```python
from build123d import *

# Parameters (mm, degrees)
SKETCH1_W           = 152.4
SKETCH1_H           = 69.85
BOSS_EXTRUDE1_DEPTH = 19.05
CUT_EXTRUDE1_DEPTH  = 7.1374
CUT_EXTRUDE2_REACH  = 71.85
SKETCH3_R           = 4.0132


with BuildPart() as part:
    # Sketch1 → Boss-Extrude1 (new body)
    with BuildSketch(Plane.XY):
        Rectangle(SKETCH1_W, SKETCH1_H)
    extrude(amount=BOSS_EXTRUDE1_DEPTH)

    # Sketch2 → Cut-Extrude1 (cut)
    with BuildSketch(Plane.XY.offset(19.05)):
        with BuildLine():
            Line((-45.24375, 28.575), (-30.95625, 28.575))
            ThreePointArc((-30.95625, 28.575), (-27.588653955, 27.180096045), (-26.19375, 23.8125))
            Line((-26.19375, 23.8125), (-26.19375, -23.8125))
            ThreePointArc((-26.19375, -23.8125), (-27.588653955, -27.180096045), (-30.95625, -28.575))
            Line((-30.95625, -28.575), (-45.24375, -28.575))
            ThreePointArc((-45.24375, -28.575), (-48.611346045, -27.180096045), (-50.00625, -23.8125))
            Line((-50.00625, -23.8125), (-50.00625, 23.8125))
            ThreePointArc((-50.00625, 23.8125), (-48.611346045, 27.180096045), (-45.24375, 28.575))
        make_face()
        with BuildLine():
            Line((7.14375, 28.575), (-7.14375, 28.575))
            ThreePointArc((-7.14375, 28.575), (-10.511346045, 27.180096045), (-11.90625, 23.8125))
            Line((-11.90625, 23.8125), (-11.90625, -23.8125))
            ThreePointArc((-11.90625, -23.8125), (-10.511346045, -27.180096045), (-7.14375, -28.575))
            Line((-7.14375, -28.575), (7.14375, -28.575))
            ThreePointArc((7.14375, -28.575), (10.511346045, -27.180096045), (11.90625, -23.8125))
            Line((11.90625, -23.8125), (11.90625, 23.8125))
            ThreePointArc((11.90625, 23.8125), (10.511346045, 27.180096045), (7.14375, 28.575))
        make_face()
        with BuildLine():
            Line((30.95625, 28.575), (45.24375, 28.575))
            ThreePointArc((45.24375, 28.575), (48.611346045, 27.180096045), (50.00625, 23.8125))
            Line((50.00625, 23.8125), (50.00625, -23.8125))
            ThreePointArc((50.00625, -23.8125), (48.611346045, -27.180096045), (45.24375, -28.575))
            Line((45.24375, -28.575), (30.95625, -28.575))
            ThreePointArc((30.95625, -28.575), (27.588653955, -27.180096045), (26.19375, -23.8125))
            Line((26.19375, -23.8125), (26.19375, 23.8125))
            ThreePointArc((26.19375, 23.8125), (27.588653955, 27.180096045), (30.95625, 28.575))
        make_face()
        with BuildLine():
            Line((-69.85, 28.575), (-66.675, 28.575))
            ThreePointArc((-66.675, 28.575), (-64.42993597, 27.64506403), (-63.5, 25.4))
            Line((-63.5, 25.4), (-63.5, -25.4))
            ThreePointArc((-63.5, -25.4), (-64.42993597, -27.64506403), (-66.675, -28.575))
            Line((-66.675, -28.575), (-69.85, -28.575))
            ThreePointArc((-69.85, -28.575), (-72.09506403, -27.64506403), (-73.025, -25.4))
            Line((-73.025, -25.4), (-73.025, 25.4))
            ThreePointArc((-73.025, 25.4), (-72.09506403, 27.64506403), (-69.85, 28.575))
        make_face()
        with BuildLine():
            Line((66.675, 28.575), (69.85, 28.575))
            ThreePointArc((69.85, 28.575), (72.09506403, 27.64506403), (73.025, 25.4))
            Line((73.025, 25.4), (73.025, -25.4))
            ThreePointArc((73.025, -25.4), (72.09506403, -27.64506403), (69.85, -28.575))
            Line((69.85, -28.575), (66.675, -28.575))
            ThreePointArc((66.675, -28.575), (64.42993597, -27.64506403), (63.5, -25.4))
            Line((63.5, -25.4), (63.5, 25.4))
            ThreePointArc((63.5, 25.4), (64.42993597, 27.64506403), (66.675, 28.575))
        make_face()
    extrude(amount=-CUT_EXTRUDE1_DEPTH, mode=Mode.SUBTRACT)

    # Sketch3 → Cut-Extrude2 (cut, up to next)
    with BuildSketch(Plane(origin=(0, 34.925, 0), x_dir=(1, 0, 0), z_dir=(0, 1, 0)), mode=Mode.PRIVATE) as cut_extrude2_sk1:
        with Locations(Location((-57.15, -9.525, 0), (0, 0, 270))):  # turned: the seam where the file's is
            Circle(SKETCH3_R)
    cut_extrude2_tool1 = extrude(cut_extrude2_sk1.sketch, amount=-CUT_EXTRUDE2_REACH, mode=Mode.PRIVATE) & part.part
    add(cut_extrude2_tool1.solids().sort_by_distance((-57.15, 34.925, 9.525))[0], mode=Mode.SUBTRACT)
    # Sketch3 → Cut-Extrude2 (cut, up to next)
    with BuildSketch(Plane(origin=(0, 34.925, 0), x_dir=(1, 0, 0), z_dir=(0, 1, 0)), mode=Mode.PRIVATE) as cut_extrude2_sk2:
        with Locations(Location((-19.05, -9.525, 0), (0, 0, 270))):  # turned: the seam where the file's is
            Circle(SKETCH3_R)
    cut_extrude2_tool2 = extrude(cut_extrude2_sk2.sketch, amount=-CUT_EXTRUDE2_REACH, mode=Mode.PRIVATE) & part.part
    add(cut_extrude2_tool2.solids().sort_by_distance((-19.05, 34.925, 9.525))[0], mode=Mode.SUBTRACT)
    # Sketch3 → Cut-Extrude2 (cut, up to next)
    with BuildSketch(Plane(origin=(0, 34.925, 0), x_dir=(1, 0, 0), z_dir=(0, 1, 0)), mode=Mode.PRIVATE) as cut_extrude2_sk3:
        with Locations(Location((19.05, -9.525, 0), (0, 0, 270))):  # turned: the seam where the file's is
            Circle(SKETCH3_R)
    cut_extrude2_tool3 = extrude(cut_extrude2_sk3.sketch, amount=-CUT_EXTRUDE2_REACH, mode=Mode.PRIVATE) & part.part
    add(cut_extrude2_tool3.solids().sort_by_distance((19.05, 34.925, 9.525))[0], mode=Mode.SUBTRACT)
    # Sketch3 → Cut-Extrude2 (cut, up to next)
    with BuildSketch(Plane(origin=(0, 34.925, 0), x_dir=(1, 0, 0), z_dir=(0, 1, 0)), mode=Mode.PRIVATE) as cut_extrude2_sk4:
        with Locations(Location((57.15, -9.525, 0), (0, 0, 270))):  # turned: the seam where the file's is
            Circle(SKETCH3_R)
    cut_extrude2_tool4 = extrude(cut_extrude2_sk4.sketch, amount=-CUT_EXTRUDE2_REACH, mode=Mode.PRIVATE) & part.part
    add(cut_extrude2_tool4.solids().sort_by_distance((57.15, 34.925, 9.525))[0], mode=Mode.SUBTRACT)


solid = part.part
```
Can you work these out from the model? Positions are in its coordinate system, mm. A direction names the side the tool comes from. Coordinates: 2 decimals unless noted, no trailing zeros. Write each loop counter-clockwise with the first axis right and the second up, starting at its lowest first coordinate (ties: lowest second). Pieces come first, ordered by that corner, then holes. Notation, with made-up numbers: M 18,35 L 44,35 A15 cw 44,60 Z; hole C 36,16 d10. An arc over 180 degrees is marked long. Write item = value, one per line. Start each with the question number.
Q1. If we section it at B-B, the plane x = 57.15: Write out the boundary of the cut face in (y, z) (3 decimals), then the cut area to 3 significant figures.
Q2. On a 3-axis mill with a long thin cutter (end or side, diameter ignored), from which of +Z, -Z, +X, -X, +Y, -Y can I reach the whole of each face in a straight line? I mean faces 1 (the face through (-60.7, 0.5, 11.4)), 2 (the face through (50.006, 0, 16)). Say none if no direction works.
Q3. Thinking about a two-plate mould opening in X: for faces 3 (the face through (10.55, 27.14, 15.53)), 4 (the face through (-76.2, 0, 9)), 5 (the face through (-1, -34.925, 9)), which applies, released by +X, released by -X, zero draft, split by the parting line, or undercut?
Q4. I'm going to push flat-ended pins straight in: pin 1 (3 mm diameter, centred on x = -33, y = -2, fed in from +Z); pin 2 (3 mm diameter, centred on x = -19.5, y = 23, fed in from -Z). Where does each tip first touch, or does it pass through?
Q5. If we section it at A-A, the plane y = 15.5: Write out the boundary of the cut face in (x, z) (3 decimals), then the cut area to 3 significant figures.
Q6. If I drill on L1, parallel to X at y = 20.5, z = 16.5 (3 decimals); L2, parallel to Z at x = -19, y = -8; L3, parallel to X at y = -15, z = 6.5, over which ranges is the centre line in solid material (lowest first)? Write a range as [from, to].
Q7. If we section it at C-C, the plane z = 8.5: Write out the boundary of the cut face in (x, y) (3 decimals), then the cut area to 3 significant figures.
Q8. If we section it at D-D, the plane z = 17.25: State how many separate pieces and enclosed holes the cut face has, then the cut area to 3 significant figures.
Check sheet entries:
q1.outline = M -34.925,0 L 34.925,0 L 34.925,5.512 L -34.925,5.512 Z; M -34.925,13.538 L 34.925,13.538 L 34.925,19.05 L -34.925,19.05 Z
q1.area = 770 mm²
q2.face_1 = +Y, -Y
q2.face_2 = +Z
q3.face_3 = undercut
q3.face_4 = released by -X
q3.face_5 = zero draft
q4.pin_1 = 11.91
q4.pin_2 = 0
q5.outline = M -76.2,0 L 76.2,0 L 76.2,19.05 L 73.025,19.05 L 73.025,11.913 L 63.5,11.913 L 63.5,19.05 L 50.006,19.05 L 50.006,11.913 L 26.194,11.913 L 26.194,19.05 L 11.906,19.05 L 11.906,11.913 L -11.906,11.913 L -11.906,19.05 L -26.194,19.05 L -26.194,11.913 L -50.006,11.913 L -50.006,19.05 L -63.5,19.05 L -63.5,11.913 L -73.025,11.913 L -73.025,19.05 L -76.2,19.05 Z; hole C -57.15,9.525 d8.026; hole C -19.05,9.525 d8.026; hole C 19.05,9.525 d8.026; hole C 57.15,9.525 d8.026
q5.area = 2,050 mm²
q6.L1 = [-76.2, -73.025], [-63.5, -50.006], [-26.194, -11.906], [11.906, 26.194], [50.006, 63.5], [73.025, 76.2]
q6.L2 = [0, 5.51], [13.54, 19.05]
q6.L3 = [-76.2, -59.79], [-54.51, -21.69], [-16.41, 16.41], [21.69, 54.51], [59.79, 76.2]
q7.outline = M -76.2,-34.925 L -61.03,-34.925 L -61.03,34.925 L -76.2,34.925 Z; M -53.27,-34.925 L -22.93,-34.925 L -22.93,34.925 L -53.27,34.925 Z; M -15.17,-34.925 L 15.17,-34.925 L 15.17,34.925 L -15.17,34.925 Z; M 22.93,-34.925 L 53.27,-34.925 L 53.27,34.925 L 22.93,34.925 Z; M 61.03,-34.925 L 76.2,-34.925 L 76.2,34.925 L 61.03,34.925 Z
q7.area = 8,480 mm²
q8.separate_pieces = 1
q8.enclosed_holes = 5
q8.area = 5,550 mm²
